Verification items for the finished model (mm, model axes). A direction names the side the tool comes from. Coordinates: 2 decimals unless noted, no trailing zeros. Order: outer loops, then holes, each group sorted by start corner. A loop starts at its lowest first (then second) coordinate and runs counter-clockwise, first axis right, second up. Notation, with made-up numbers: (-26, 35.5) -> (18, 35.5) arc R16 ccw to (18, 48.5) -> close; hole circle Ø1 at (17, 43). An arc over 180 degrees is marked (long way). Write each question's results on one line, items separated by ' | '. Start each with the question number.
(1) Set-up check for faces 4 (the flat face through (6, 3, 40.5)), 5 (the flat face through (6.02, 11, 2)), 6 (the flat face through (9, 11, 31)), 7 (the flat face through (6, 3.5, 3)): record each of +Z, -Z, +X, -X, +Y, -Y from which the full face is reachable in a straight line by a thin tool's end or side.
(2) Cross-section at C-C on y = 4.5. Enter the section's corners in (x, z) (3 decimals).
(3) Go/stop test with flat-tipped pins: pin 1 (3.5 mm diameter, centred on x = 7.5, y = -0.5, fed in from -Z); pin 2 (5 mm diameter, centred on x = 2.5, z = -22.265, fed in from -Y); pin 3 (3 mm diameter, centred on y = 10.5, z = -6, fed in from -X). Record where each tip stops, or that it passes through.
(4) Cross-section at A-A on z = -15. Enter the section's corners in (x, y).
(5) Draft check along Z on faces 1 (the cylindrical face through (10.11, 8.57, 19.01)), 2 (the flat face through (6, 3, -35.5)), 3 (the flat face through (6, -3.5, 38)). Enter one of: +Z half, -Z half, draft (parallel to the pull), parting line (faces both ways), or undercut.
(6) Thickness scan on probe 1 along Z at (x, y) = (9, 10.25); probe 2 along Z at (x, y) = (10.5, -2); probe 3 along Z at (x, y) = (7.75, 11.5). Record the ranges inside material, lowest first. Write a range as [from, to].
(7) Cross-section at D-D on z = 13. Enter the section's corners in (x, y).
(8) Cross-section at B-B on x = 2.5. Enter the section's corners in (y, z) (3 decimals).
```python
from build123d import *

# Parameters (mm, degrees)
F1_DEPTH  = 12
F2_W      = 6.02
F2_H      = 5
F3_DEPTH  = 76
F4_R      = 1.5
F5_DEPTH  = 25
F6_R      = 1.5
F7_DEPTH  = 25
F8_W      = 12
F8_H      = 5
F9_DEPTH  = 7
F10_R     = 2
F11_DEPTH = 76
F12_W     = 5.98
F12_H     = 9.5
F12_H_2   = 7.5
F13_DEPTH = 5
F14_R     = 1.5
F15_DEPTH = 25


# Not quite as in the source:
# - a feature names something its author has since deleted; it is built from what else it names


with BuildPart() as f1:
    # F0 (on Right) → F1 (new body)
    with BuildSketch(Plane.YZ):
        Polygon((13.5, 40.5), (-3.5, 40.5), (-3.5, 35.5), (3.5, 35.5), (3.5, -35.5), (13.5, -35.5), align=None)
    extrude(amount=F1_DEPTH)

    # F2 (on face) → F3 (cut)
    with BuildSketch(Plane.XY.offset(40.5)):
        with Locations((3.01, 11)):
            Rectangle(F2_W, F2_H)
    extrude(amount=-F3_DEPTH, mode=Mode.SUBTRACT)

    # F4 (on face) → F5 (cut)
    with BuildSketch(Plane(origin=(0, 13.5, 0), x_dir=(-1, 0, 0), z_dir=(0, 1, 0))):
        with Locations((-9, 28.5)):
            Circle(F4_R)
        with Locations((-9, -23.5)):
            Circle(F4_R)
    extrude(amount=-F5_DEPTH, mode=Mode.SUBTRACT)

    # F6 (on face) → F7 (cut)
    with BuildSketch(Plane(origin=(0, 8.5, 0), x_dir=(-1, 0, 0), z_dir=(0, 1, 0))):
        with Locations((-2.5, -22.265)):
            Circle(F6_R)
        with Locations((-2.5, 27.265)):
            Circle(F6_R)
    extrude(amount=-F7_DEPTH, mode=Mode.SUBTRACT)

    # F8 (on face) → F9 (join)
    with BuildSketch(Plane.XZ.offset(-3.5)):
        with Locations((6, -33)):
            Rectangle(F8_W, F8_H)
    extrude(amount=F9_DEPTH)

    # F10 (on face) → F11 (cut)
    with BuildSketch(Plane.XY.offset(40.5)):
        with Locations((7, 0.5)):
            Circle(F10_R)
    extrude(amount=-F11_DEPTH, mode=Mode.SUBTRACT)

    # F12 (on face) → F13 (cut)
    with BuildSketch(Plane(origin=(0, 13.5, 0), x_dir=(-1, 0, 0), z_dir=(0, 1, 0))):
        with Locations((-9.01, 35.75)):
            Rectangle(F12_W, F12_H)
        with Locations((-9.01, -31.75)):
            Rectangle(F12_W, F12_H_2)
    extrude(amount=-F13_DEPTH, mode=Mode.SUBTRACT)

    # F14 (on face) → F15 (cut)
    with BuildSketch(Plane(origin=(0, 13.5, 0), x_dir=(-1, 0, 0), z_dir=(0, 1, 0))):
        with Locations((-9, -15)):
            Circle(F14_R)
        with Locations((-9, 18)):
            Circle(F14_R)
    extrude(amount=-F15_DEPTH, mode=Mode.SUBTRACT)


solid = f1.part
```
Results are:
1) face 4: +Z, +X, -X, +Y, -Y | face 5: +Z, -Z, -X, +Y | face 6: +Z, +X, -X, +Y | face 7: +X, -X, -Y
2) outline: (0, -35.5) -> (12, -35.5) -> (12, 40.5) -> (0, 40.5) -> close; hole circle Ø3 at (2.5, -22.265); hole circle Ø3 at (2.5, 27.265); hole circle Ø3 at (9, -23.5); hole circle Ø3 at (9, -15); hole circle Ø3 at (9, 18); hole circle Ø3 at (9, 28.5)
3) pin 1: stops at z = -35.5 | pin 2: stops at y = 3.5 | pin 3: stops at x = 6.02
4) outline: (0, 3.5) -> (7.5, 3.5) -> (7.5, 13.5) -> (6.02, 13.5) -> (6.02, 8.5) -> (0, 8.5) -> close; (10.5, 3.5) -> (12, 3.5) -> (12, 13.5) -> (10.5, 13.5) -> close
5) face 1: undercut | face 2: -Z half | face 3: draft
6) probe 1: z = [-28, -25], [-22, -16.5], [-13.5, 16.5], [19.5, 27], [30, 31] | probe 2: z = [-35.5, -30.5], [35.5, 40.5] | probe 3: z = [-28, -24.33], [-22.67, -15.83], [-14.17, 17.17], [18.83, 27.67], [29.33, 31]
7) outline: (0, 3.5) -> (12, 3.5) -> (12, 13.5) -> (6.02, 13.5) -> (6.02, 8.5) -> (0, 8.5) -> close
8) outline: (-3.5, -35.5) -> (8.5, -35.5) -> (8.5, -23.765) -> (3.5, -23.765) -> (3.5, -30.5) -> (-3.5, -30.5) -> close; (-3.5, 35.5) -> (3.5, 35.5) -> (3.5, 28.765) -> (8.5, 28.765) -> (8.5, 40.5) -> (-3.5, 40.5) -> close; (3.5, -20.765) -> (8.5, -20.765) -> (8.5, 25.765) -> (3.5, 25.765) -> close
